Check sheet for the modelled part. Datum: model origin and axes. Units: mm. A direction names the side the tool comes from. Coordinates: 2 decimals unless noted, no trailing zeros. Loops run counter-clockwise (first coordinate to the right, second up) from the corner with the lowest first, then second, coordinate; pieces in that order, holes last. Notation, with made-up numbers: (-17, 34.25) - (10, 34.25) arc R28 ccw to (10, 52.25) - close; hole circle Ø11 at (-24.5, 63). An arc over 180 degrees is marked (long way). Use a Markdown table: item, result. Add a question column.
1) Sectioned sample at C-C, the plane x = 6.25. Enter the section's corners in (y, z).
2) Draft check along X on faces 5 (the cylindrical face through (3.03, 1.13, -0.25)), 6 (the flat face through (-0.635, 0, 0)), 7 (the cylindrical face through (6.4, 0.1, -7.5)), 8 (the flat face through (6.121, 0, -3)). Enter one of: pulls with the +X half, pulls with the -X half, needs draft (parallel to the pull), parting line crosses it, or undercut.
3) Sectioned sample at D-D, the plane y = -1.7. Enter the section's corners in (x, z), then the cut area to 3 significant figures.
4) Sectioned sample at B-B, the plane z = 1.5. Enter the section's corners in (x, y), then the cut area to 3 significant figures.
5) Tool access check on faces 1 (the cylindrical face through (6.44, -0.7, -0.92)), 2 (the flat face through (0.737, 0, -3)), 3 (the flat face through (-0.635, 0, -6)), 4 (the cylindrical face through (-0.3, 0.1, -7.5)). Record the directions out of +Z, -Z, +X, -X, +Y, -Y that give a thin tool (end or side, any length) a straight path to the whole face; none if there is none.
6) Go/stop test with flat-tipped pins: P1, Ø3, axis at x = 5.5, z = -1, coming from the -Y side; P2, Ø1, axis at x = 1.5, z = -1, coming from the +Y side; P3, Ø3, axis at x = 3, y = -2, coming from the +Z side. Record where each tip stops, or that it passes through.
7) Thickness scan on line 1 (X direction, y = -1.35, z = -7.25); line 2 (Z direction, x = 6.25, y = 0.8); line 3 (Z direction, x = 4, y = 0.55). Record the ranges inside material, lowest first.
from build123d import *

# Parameters (mm, degrees)
BOSS_EXTRUDE1_DEPTH = 0.7366
SKETCH2_R           = 1.1557
BOSS_EXTRUDE2_DEPTH = 4.6482
BOSS_EXTRUDE3_START = 0.635
SKETCH3_R           = 1.1557
BOSS_EXTRUDE3_DEPTH = 0.635


with BuildPart() as part:
    # Sketch1 → Boss-Extrude1 (new body)
    with BuildSketch(Plane(origin=(0, 0, 0), x_dir=(0, 0, -1), z_dir=(1, 0, 0))):
        with BuildLine():
            ThreePointArc((1.5875, 2.482159687), (-2.9464, 0), (1.5875, -2.482159687))
            ThreePointArc((1.5875, -2.482159687), (3.175, -2.017919373), (4.7625, -2.482159687))
            ThreePointArc((4.7625, -2.482159687), (9.2964, 0), (4.7625, 2.482159687))
            ThreePointArc((4.7625, 2.482159687), (3.175, 2.017919373), (1.5875, 2.482159687))
        make_face()
    boss_extrude1 = extrude(amount=BOSS_EXTRUDE1_DEPTH)

    # Sketch2 → Boss-Extrude2 (add)
    with BuildSketch(Plane(origin=(0.7366, 0, 0), x_dir=(0, 0, -1), z_dir=(1, 0, 0))):
        with Locations(Location((0, 0, 0), (0, 0, 180))):
            Circle(SKETCH2_R)
        with Locations(Location((6.35, 0, 0), (0, 0, 180))):
            Circle(SKETCH2_R)
    extrude(amount=BOSS_EXTRUDE2_DEPTH)

    # Sketch3 → Boss-Extrude3 (add)
    with BuildSketch(Plane.ZY.offset(BOSS_EXTRUDE3_START)):
        Circle(SKETCH3_R)
        with Locations((-6.35, 0)):
            Circle(SKETCH3_R)
    boss_extrude3 = extrude(amount=-BOSS_EXTRUDE3_DEPTH)

    # Mirror1: Boss-Extrude1, Boss-Extrude3 across plane
    add(boss_extrude1.mirror(Plane(origin=(3.0607, 0, 0), x_dir=(0, 0, 1), z_dir=(1, 0, 0))))
    add(boss_extrude3.mirror(Plane(origin=(3.0607, 0, 0), x_dir=(0, 0, 1), z_dir=(1, 0, 0))))


solid = part.part
Solved:
| question | item | result |
|---|---|---|
| 1 | outline | circle Ø2.31 at (0, -6.35); circle Ø2.31 at (0, 0) |
| 2 | face 5 | undercut |
| 2 | face 6 | pulls with the -X half |
| 2 | face 7 | needs draft |
| 2 | face 8 | pulls with the +X half |
| 3 | outline | (0, -8.76) - (0.74, -8.76) - (0.74, 2.41) - (0, 2.41) - close; (5.38, -8.76) - (6.12, -8.76) - (6.12, 2.41) - (5.38, 2.41) - close |
| 3 | area | 16.4 mm2 |
| 4 | outline | (0, -2.54) - (0.74, -2.54) - (0.74, 2.54) - (0, 2.54) - close; (5.38, -2.54) - (6.12, -2.54) - (6.12, 2.54) - (5.38, 2.54) - close |
| 4 | area | 7.47 mm2 |
| 5 | face 1 | +X |
| 5 | face 2 | none |
| 5 | face 3 | +Z, -Z, -X, +Y, -Y |
| 5 | face 4 | -X |
| 6 | P1 | stops at y = -2.95 |
| 6 | P2 | stops at y = 1.04 |
| 6 | P3 | stops at z = 1.04 |
| 7 | line 1 | x = 0 to 0.74, 5.38 to 6.12 |
| 7 | line 2 | z = -7.18 to -5.52, -0.83 to 0.83 |
| 7 | line 3 | z = -7.37 to -5.33, -1.02 to 1.02 |
